Can you work these out from the model? Positions are in its coordinate system, mm. Round coordinates to 2 decimals unless told otherwise and drop trailing zeros. Write each loop counter-clockwise with the first axis right and the second up, starting at its lowest first coordinate (ties: lowest second). Pieces come first, ordered by that corner, then holes. Notation, with made-up numbers: (73, 5) -> (98, 5) arc R35 cw to (98, 39) -> close; hole circle Ø11 at (87.5, 24.25). An arc over 180 degrees is marked (long way). Write item = value, one per line. Start each with the question number.
1) Thinking about a two-plate mould opening in Z: for faces 1 (the face through (192, 46, 0)), 2 (the face through (192, 46, 5)), which applies, +Z half, -Z half, draft (parallel to the pull), parting line (faces both ways), or undercut?
2) Imagine slicing it at B-B, the plane z = 2.5. State how many separate pieces and enclosed holes the cut face has, then the cut area to 3 significant figures.
3) I'm going to push flat-ended pins straight in: pin 1 (2 mm diameter, centred on x = 35, z = 3, fed in from -Y); pin 2 (1.2 mm diameter, centred on y = 45, z = 2.5, fed in from +X); pin 3 (1.5 mm diameter, centred on x = 355, z = 2.5, fed in from -Y); pin 4 (2 mm diameter, centred on y = 45, z = 2.5, fed in from -X). Where does each tip first touch, or does it pass through?
4) If I drill on line 1 (X direction, y = 6, z = 2.5); line 2 (X direction, y = 51, z = 0.3); line 3 (Y direction, x = 379.5, z = 2.5), over which ranges is the centre line in solid material (lowest first)?
5) Imagine slicing it at A-A, the plane x = 82. Please give me the cut outline in (y, z).
from build123d import *

# Parameters (mm, degrees)
SKETCH1_W           = 390
SKETCH1_H           = 90
BOSS_EXTRUDE2_DEPTH = 5
SKETCH2_R           = 1.25
CUT_EXTRUDE1_DEPTH  = 15
CUT_EXTRUDE2_START  = -15
SKETCH3_R           = 1.25
CUT_EXTRUDE2_DEPTH  = 15
SKETCH4_R           = 1.25
CUT_EXTRUDE3_DEPTH  = 15


with BuildPart() as part:
    # Sketch1 → Boss-Extrude2 (new body)
    with BuildSketch(Plane.XY):
        with Locations((195, 45)):
            Rectangle(SKETCH1_W, SKETCH1_H)
        with BuildLine():
            Line((41, 60), (59, 60))
            ThreePointArc((59, 60), (59.707106781, 59.707106781), (60, 59))
            Line((60, 59), (60, 48))
            ThreePointArc((60, 48), (59.707106781, 47.292893219), (59, 47))
            Line((59, 47), (41, 47))
            ThreePointArc((41, 47), (40.292893219, 47.292893219), (40, 48))
            Line((40, 48), (40, 59))
            ThreePointArc((40, 59), (40.292893219, 59.707106781), (41, 60))
        make_face(mode=Mode.SUBTRACT)
        with BuildLine():
            Line((76, 60), (94, 60))
            ThreePointArc((94, 60), (94.707106781, 59.707106781), (95, 59))
            Line((95, 59), (95, 48))
            ThreePointArc((95, 48), (94.707106781, 47.292893219), (94, 47))
            Line((94, 47), (76, 47))
            ThreePointArc((76, 47), (75.292893219, 47.292893219), (75, 48))
            Line((75, 48), (75, 59))
            ThreePointArc((75, 59), (75.292893219, 59.707106781), (76, 60))
        make_face(mode=Mode.SUBTRACT)
    extrude(amount=BOSS_EXTRUDE2_DEPTH)

    # Sketch2 → Cut-Extrude1 (cut)
    with BuildSketch(Plane.ZY):
        with Locations((2.5, 45)):
            Circle(SKETCH2_R)
    extrude(amount=-CUT_EXTRUDE1_DEPTH, mode=Mode.SUBTRACT)

    # Sketch3 → Cut-Extrude2 (cut)
    with BuildSketch(Plane(origin=(390, 0, 0), x_dir=(0, 0, -1), z_dir=(1, 0, 0)).offset(CUT_EXTRUDE2_START)):
        with Locations(Location((-2.5, 45, 0), (0, 0, 180))):
            Circle(SKETCH3_R)
    extrude(amount=CUT_EXTRUDE2_DEPTH, mode=Mode.SUBTRACT)

    # Sketch4 → Cut-Extrude3 (cut)
    with BuildSketch(Plane.XZ):
        with Locations(Location((35, 2.5, 0), (0, 0, 270))):
            Circle(SKETCH4_R)
        with Locations(Location((355, 2.5, 0), (0, 0, 270))):
            Circle(SKETCH4_R)
    extrude(amount=-CUT_EXTRUDE3_DEPTH, mode=Mode.SUBTRACT)


solid = part.part
Reported:
q1.face_1 = -Z half
q1.face_2 = +Z half
q2.separate_pieces = 1
q2.enclosed_holes = 2
q2.area = 34,400 mm²
q3.pin_1 = 0
q3.pin_2 = 375
q3.pin_3 = 15
q3.pin_4 = 15
q4.line_1 = 0 to 33.75, 36.25 to 353.75, 356.25 to 390
q4.line_2 = 0 to 40, 60 to 75, 95 to 390
q4.line_3 = 0 to 43.75, 46.25 to 90
q5.outline = (0, 0) -> (47, 0) -> (47, 5) -> (0, 5) -> close; (60, 0) -> (90, 0) -> (90, 5) -> (60, 5) -> close
